Can you work these out from the model? Positions are in its coordinate system, mm. Face numbers are marked on the shaded views. A direction names the side the tool comes from. Give positions to 0.01 mm unless a question says otherwise; leave off trailing zeros. Loops run counter-clockwise (first coordinate to the right, second up) from the corner with the lowest first, then second, coordinate; pieces in that order, holes last. Notation, with made-up numbers: (30, 72) -> (86, 72) arc R28 ccw to (86, 107) -> close; hole circle Ø6 at (19.5, 47.5). An arc over 180 degrees is marked (long way). Return JSON: item names as keys, results as strings. Group by question number.
Q1. Suppose I cut it at C-C, the plane x = -4.5. Please give me the cut outline in (y, z).
Q2. Which directions (+Z, -Z, +X, -X, +Y, -Y) give clear straight access to the entire face, cutting with the end or side of a thin tool? Please do the marked faces 1 and 2.
Q3. Suppose I cut it at B-B, the plane y = -1.5. Please give me the cut outline in (x, z).
Q4. Suppose I cut it at D-D, the plane z = 16.25. Please give me the cut outline in (x, y) (3 decimals), and give its area (3 significant figures).
Q5. Suppose I cut it at A-A, the plane z = 18.5. Please give me the cut outline in (x, y).
Q6. Will these pins go through, and if not, where does the flat tip stop? pin 1 (9 mm diameter, centred on y = -0.5, z = 13.5, fed in from +X); pin 2 (5.5 mm diameter, centred on x = 1.5, y = -1.5, fed in from +Z); pin 3 (1.5 mm diameter, centred on y = -1.5, z = 15, fed in from +X); pin 4 (3 mm diameter, centred on y = 7, z = 8.5, fed in from -X).
Q7. I need wall thicknesses on line 1 along X through (y, z) = (-5, 14.5); line 2 along X through (y, z) = (-6.75, 12); line 3 along X through (y, z) = (-7.25, 6.5). Which ranges of each line are inside material? Lowest first, please. Write a range as [from, to].
Autodesk Inventor part; units mm, degrees
ref_plane "YZ Plane" through (0, 0, 0) normal (1, 0, 0) x (0, 1, 0)
ref_plane "XZ Plane" through (0, 0, 0) normal (0, 1, 0) x (-1, 0, 0)
ref_plane "XY Plane" through (0, 0, 0) normal (0, 0, 1) x (1, 0, 0)
sketch "草图2" plane through (0, 0, 0) normal (0, 1, 0) x (-1, 0, 0)
  line L0 (-18, 0) -> (18, 0)
  line L1 (18, 0) -> (18, 5)
  line L2 (18, 5) -> (-18, 5)
  line L3 (-18, 5) -> (-18, 0)
  line L4 (-18, 5) -> (-11, 20)
  line L5 (-11, 20) -> (-3.5, 20)
  line L6 (-3.5, 20) -> (-3.5, 9)
  line L7 (-3.5, 9) -> (3.5, 9)
  line L8 (3.5, 9) -> (3.5, 20)
  line L9 (3.5, 20) -> (11, 20)
  line L10 (11, 20) -> (18, 5)
  point P0 (0, 0)
  point P1 (0, 0)
  point P2 (0, 5)
  point P3 (0, 9)
  dimension "d0" = 36
  dimension "d1" = 5
  dimension "d2" = 20
  dimension "d3" = 11
  dimension "d4" = 7
  dimension "d5" = 22
extrude "拉伸1" add sketch "草图2" along normal mid plane 22 contours L3 L2 L1 L0
extrude "拉伸2" add sketch "草图2" along normal mid plane 22 contours L4 L5 L6 L7 L8 L9 L10 L2
sketch "草图3" plane through (18, -11, 0) normal (1, 0, 0) x (0, 0, -1)
  line L0 (-5, 22) -> (-5, 0)
  line L1 (-20, 22) -> (-5, 22)
  line L2 (-20, 0) -> (-20, 22)
  line L3 (-5, 0) -> (-20, 0)
  line L4 (0, 0) -> (0, 22)
  line L5 (-5, 22) -> (0, 22)
  line L6 (-5, 22) -> (-5, 0)
  line L7 (0, 0) -> (-5, 0)
  line L8 (-5, 0) -> (-20, 5.5)
  line L9 (-5, 22) -> (-20, 16.5)
  line L10 (-20, 0) -> (-20, 22)
  line L11 (-20, 16.5) -> (-20, 5.5)
  line L12 (-5, 0) -> (-5, 22)
  line L13 (-5, 0) -> (-5, 22)
  line L14 (-5, 0) -> (0, 0)
  line L15 (0, 0) -> (0, 22)
  line L16 (0, 22) -> (0, 0)
  line L17 (-5, 22) -> (0, 22)
  line L18 (-5, 22) -> (0, 22)
  point P0 (0, 11)
  dimension "d10" = 11
extrude "拉伸3" cut sketch "草图3" against normal blind 36 contours L5 L4 L7 L0 | L0 L8 L2 L9 keep common part
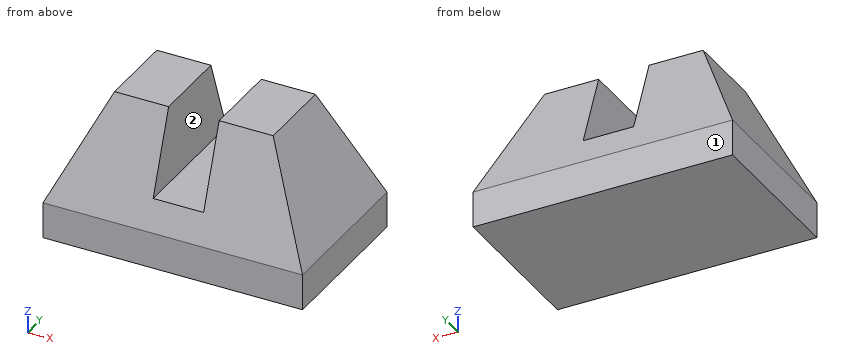
Ans:
{
 "1": {"outline": "(-11, 0) -> (11, 0) -> (11, 5) -> (5.5, 20) -> (-5.5, 20) -> (-11, 5) -> close"},
 "2": {"face 1": "+Z, -Z, +X, -X, +Y", "face 2": "+Z, +Y, -Y"},
 "3": {"outline": "(-18, 0) -> (18, 0) -> (18, 5) -> (11, 20) -> (3.5, 20) -> (3.5, 9) -> (-3.5, 9) -> (-3.5, 20) -> (-11, 20) -> (-18, 5) -> close"},
 "4": {"outline": "(-12.75, -6.875) -> (-3.5, -6.875) -> (-3.5, 6.875) -> (-12.75, 6.875) -> close; (3.5, -6.875) -> (12.75, -6.875) -> (12.75, 6.875) -> (3.5, 6.875) -> close", "area": "254 mm^2"},
 "5": {"outline": "(-11.7, -6.05) -> (-3.5, -6.05) -> (-3.5, 6.05) -> (-11.7, 6.05) -> close; (3.5, -6.05) -> (11.7, -6.05) -> (11.7, 6.05) -> (3.5, 6.05) -> close"},
 "6": {"pin 1": "stops at x = 16.13", "pin 2": "stops at z = 20", "pin 3": "stops at x = 13.68", "pin 4": "stops at x = -17.07"},
 "7": {"line 1": "x = [-13.57, -3.5], [3.5, 13.57]", "line 2": "x = [-14.73, -3.5], [3.5, 14.73]", "line 3": "x = [-17.3, 17.3]"}
}
